The listing builds one solid part. Answer for the finished solid, in the listing's coordinates (mm). Coordinates: 2 decimals unless noted, no trailing zeros. Write each loop counter-clockwise with the first axis right and the second up, starting at its lowest first coordinate (ties: lowest second). Pieces come first, ordered by that corner, then holes.
from build123d import *

# Parameters (mm, degrees)
SKETCH3_W           = 420
SKETCH3_H           = 170
BOSS_EXTRUDE2_DEPTH = 6
SKETCH4_W           = 6.1
SKETCH4_H           = 85
SKETCH4_W_2         = 6.2
CUT_EXTRUDE1_DEPTH  = 6
SKETCH5_R           = 2
CUT_EXTRUDE2_DEPTH  = 6
SKETCH6_W           = 6
SKETCH6_H           = 380
BOSS_EXTRUDE3_DEPTH = 30
SKETCH7_W           = 6
SKETCH7_H           = 380
CUT_EXTRUDE3_DEPTH  = 2
SKETCH8_W           = 6
SKETCH8_H           = 116.9
SKETCH8_H_2         = 133.8
BOSS_EXTRUDE4_DEPTH = 28
SKETCH9_W           = 6
SKETCH9_H           = 6.2
BOSS_EXTRUDE5_DEPTH = 113
SKETCH10_W          = 6
SKETCH10_H          = 6.2
BOSS_EXTRUDE6_DEPTH = 113
SKETCH11_W          = 6.2
SKETCH11_H          = 113
CUT_EXTRUDE4_DEPTH  = 113
SKETCH13_W          = 6
SKETCH13_H          = 28
CUT_EXTRUDE5_DEPTH  = 1000


with BuildPart() as part:
    # Sketch3 → Boss-Extrude2 (new body)
    with BuildSketch(Plane(origin=(0, 0, 0), x_dir=(0, 0, -1), z_dir=(1, 0, 0))):
        with Locations((440.911700258, 161.915861829)):
            Rectangle(SKETCH3_W, SKETCH3_H)
    extrude(amount=BOSS_EXTRUDE2_DEPTH)

    # Sketch4 → Cut-Extrude1 (cut)
    with BuildSketch(Plane(origin=(6, 0, 0), x_dir=(0, 0, -1), z_dir=(1, 0, 0))):
        with Locations((233.961700258, 119.415861829)):
            Rectangle(SKETCH4_W, SKETCH4_H)
        with Locations((647.861700258, 119.415861829)):
            Rectangle(SKETCH4_W, SKETCH4_H)
        with Locations((370.911700258, 204.415861829)):
            Rectangle(SKETCH4_W_2, SKETCH4_H)
        with Locations((510.911700258, 204.415861829)):
            Rectangle(SKETCH4_W_2, SKETCH4_H)
    extrude(amount=-CUT_EXTRUDE1_DEPTH, mode=Mode.SUBTRACT)

    # Sketch5 → Cut-Extrude2 (cut)
    with BuildSketch(Plane(origin=(6, 0, 0), x_dir=(0, 0, -1), z_dir=(1, 0, 0))):
        with Locations((299.361700258, 206.915861829)):
            Circle(SKETCH5_R)
        with Locations((299.361700258, 116.915861829)):
            Circle(SKETCH5_R)
        with Locations((440.911700258, 206.915861829)):
            Circle(SKETCH5_R)
        with Locations((582.461700258, 206.915861829)):
            Circle(SKETCH5_R)
        with Locations((582.461700258, 116.915861829)):
            Circle(SKETCH5_R)
        with Locations((440.911700258, 116.915861829)):
            Circle(SKETCH5_R)
    extrude(amount=-CUT_EXTRUDE2_DEPTH, mode=Mode.SUBTRACT)

    # Sketch6 → Boss-Extrude3 (add)
    with BuildSketch(Plane.XZ.offset(-76.915861829)):
        with Locations((3, -440.911700258)):
            Rectangle(SKETCH6_W, SKETCH6_H)
    extrude(amount=BOSS_EXTRUDE3_DEPTH)

    # Sketch7 → Cut-Extrude3 (cut)
    with BuildSketch(Plane.XZ.offset(-46.915861829)):
        with Locations((3, -440.911700258)):
            Rectangle(SKETCH7_W, SKETCH7_H)
    extrude(amount=-CUT_EXTRUDE3_DEPTH, mode=Mode.SUBTRACT)

    # Sketch8 → Boss-Extrude4 (add)
    with BuildSketch(Plane(origin=(0, 246.915861829, 0), x_dir=(1, 0, 0), z_dir=(0, 1, 0))):
        with Locations((3, 309.361700258)):
            Rectangle(SKETCH8_W, SKETCH8_H)
        with Locations((3, 572.461700258)):
            Rectangle(SKETCH8_W, SKETCH8_H)
        with Locations((3, 440.911700258)):
            Rectangle(SKETCH8_W, SKETCH8_H_2)
    extrude(amount=BOSS_EXTRUDE4_DEPTH)

    # Sketch9 → Boss-Extrude5 (add)
    with BuildSketch(Plane(origin=(0, 161.915861829, 0), x_dir=(1, 0, 0), z_dir=(0, 1, 0))):
        with Locations((3, 370.911700258)):
            Rectangle(SKETCH9_W, SKETCH9_H)
    extrude(amount=BOSS_EXTRUDE5_DEPTH)

    # Sketch10 → Boss-Extrude6 (add)
    with BuildSketch(Plane(origin=(0, 161.915861829, 0), x_dir=(1, 0, 0), z_dir=(0, 1, 0))):
        with Locations((3, 510.911700258)):
            Rectangle(SKETCH10_W, SKETCH10_H)
    extrude(amount=BOSS_EXTRUDE6_DEPTH)

    # Sketch11 → Cut-Extrude4 (cut)
    with BuildSketch(Plane(origin=(6, 0, 0), x_dir=(0, 0, -1), z_dir=(1, 0, 0))):
        with Locations((370.911700258, 105.415861829)):
            Rectangle(SKETCH11_W, SKETCH11_H)
        with Locations((510.911700258, 105.415861829)):
            Rectangle(SKETCH11_W, SKETCH11_H)
    extrude(amount=-CUT_EXTRUDE4_DEPTH, mode=Mode.SUBTRACT)

    # Sketch13 → Cut-Extrude5 (cut)
    with BuildSketch(Plane.XY.offset(-250.911700258)):
        with Locations((3, 260.915861829)):
            Rectangle(SKETCH13_W, SKETCH13_H)
        with Locations((3, 62.915861829)):
            Rectangle(SKETCH13_W, SKETCH13_H)
    extrude(amount=-CUT_EXTRUDE5_DEPTH, mode=Mode.SUBTRACT)


solid = part.part
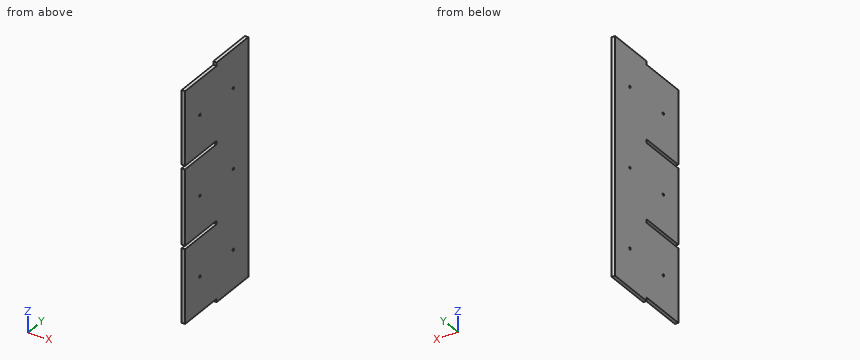
1. Flat-ended cylindrical pins translate along their axes: P1, Ø2.5, axis at y = 116.92, z = -582.46, coming from the -X side; P2, Ø3, axis at x = 2.5, y = 119.5, coming from the +Z side; P3, Ø3, axis at x = 4, z = -371.5, coming from the -Y side; P4, Ø1.8, axis at x = 2, y = 115.5, coming from the -Z side. Find the tip coordinate at first contact, or state that the pin passes through.
Results found:
P1: passes through
P2: stops at z = -237.01
P3: stops at y = 161.92
P4: stops at z = -644.81
2. Section A-A on y = 158 is taken. Give the vertices of the cut face in (x, z).
Results found:
outline: (0, -644.81) - (6, -644.81) - (6, -514.01) - (0, -514.01) - close; (0, -507.81) - (6, -507.81) - (6, -374.01) - (0, -374.01) - close; (0, -367.81) - (6, -367.81) - (6, -237.01) - (0, -237.01) - close
3. Find the intervals of material crossed by L1, parallel to Z at x = 5.4, y = 207.5; L2, parallel to Z at x = 5.45, y = 111; L3, parallel to Z at x = 4.3, y = 116.5, in increasing order.
Results found:
L1: z = -650.91 to -584.37, -580.55 to -442.82, -439 to -301.27, -297.45 to -230.91
L2: z = -644.81 to -514.01, -507.81 to -374.01, -367.81 to -237.01
L3: z = -644.81 to -584.42, -580.51 to -514.01, -507.81 to -442.87, -438.96 to -374.01, -367.81 to -301.32, -297.41 to -237.01
4. Section B-B on x = 2.4 is taken. Give the vertices of the cut face in (y, z), then the cut area to 3 significant figures.
Results found:
outline: (76.92, -644.81) - (161.92, -644.81) - (161.92, -650.91) - (246.92, -650.91) - (246.92, -230.91) - (161.92, -230.91) - (161.92, -237.01) - (76.92, -237.01) - (76.92, -367.81) - (161.92, -367.81) - (161.92, -374.01) - (76.92, -374.01) - (76.92, -507.81) - (161.92, -507.81) - (161.92, -514.01) - (76.92, -514.01) - close; hole circle Ø4 at (116.92, -582.46); hole circle Ø4 at (116.92, -440.91); hole circle Ø4 at (116.92, -299.36); hole circle Ø4 at (206.92, -582.46); hole circle Ø4 at (206.92, -440.91); hole circle Ø4 at (206.92, -299.36)
area: 69,200 mm2
